```python
from build123d import *

# Parameters (mm, degrees)
F0_W     = 19.05
F0_H     = 19.05
F0_W_2   = 12.7
F0_H_2   = 12.7
F1_DEPTH = 136.525
F2_W     = 42.5958
F2_H     = 47.244
F3_DEPTH = 9.525
F4_R     = 6.35
F5_R     = 1.5875


with BuildPart() as f1:
    # F0 (on Front) → F1 (new body)
    with BuildSketch(Plane.XZ):
        with Locations((68.0290833116, -52.153282702)):
            Rectangle(F0_W, F0_H)
        with Locations((68.0290833116, -52.153282702)):
            Rectangle(F0_W_2, F0_H_2, mode=Mode.SUBTRACT)
    extrude(amount=-F1_DEPTH)

    # F2 (on face) → F3 (join)
    with BuildSketch(Plane.XY.offset(-42.628282702)):
        with Locations((68.0290833116, 68.2625)):
            Rectangle(F2_W, F2_H)
    extrude(amount=F3_DEPTH)

    # F4
    f4_edges = [f1.edges().sort_by_distance(p)[0] for p in [
        (89.326983, 44.6405, -37.865783),
        (89.326983, 91.8845, -37.865783),
        (46.731183, 44.6405, -37.865783),
        (46.731183, 91.8845, -37.865783),
    ]]
    fillet(f4_edges, radius=F4_R)

    # F5
    f5_edges = [f1.edges().sort_by_distance(p)[0] for p in [
        (77.554083, 68.2625, -61.678283),
        (58.504083, 68.2625, -61.678283),
        (58.504083, 22.32025, -42.628283),
        (77.554083, 22.32025, -42.628283),
        (58.504083, 114.20475, -42.628283),
        (77.554083, 114.20475, -42.628283),
    ]]
    fillet(f5_edges, radius=F5_R)


solid = f1.part
```
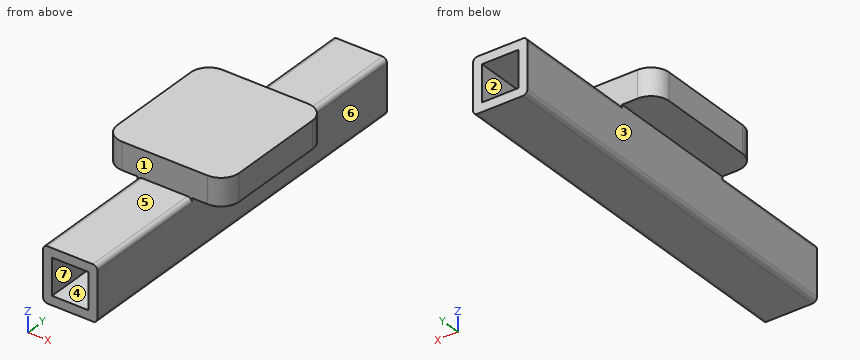
Input: part model. Units: mm. Frame: model coordinates. Face numbers are marked on the shaded views. A direction names the side the tool comes from. Give positions to 0.01 mm unless a question says otherwise; leave off trailing zeros. Order: outer loops, then holes, each group sorted by start corner. A loop starts at its lowest first (then second) coordinate and runs counter-clockwise, first axis right, second up. Notation, with made-up numbers: M -21,-21.5 L 4,-21.5 A21 cw 4,-2.5 Z; hole C 51,83.5 d2. An arc over 180 degrees is marked long. One line per question, with ' | ' between items. Start each with the question number.
1. Section query C-C (y = 124). Return the cut outline in (x, z) (1 decimal), and give its area (3 significant figures).
2. Section query B-B (z = -55.5). Return the cut outline in (x, y) (3 decimals), and give its area (3 significant figures).
3. Section query D-D (y = 61). Return the cut outline in (x, z) (1 decimal).
4. Pull-direction query (X, two-part tool) for the marked faces 1, 2, 3 and 4; classes: released by +X, released by -X, zero draft, split by the parting line, or undercut.
5. Access query for the marked faces 5, 6 and 7. Directions: +Z, -Z, +X, -X, +Y, -Y. A direction counts if a zero-diameter tool reaches every point of the face in a straight line with its end or side. Return the directions, or none.
6. Material intervals for probe 1 along X at (y, z) = (92, -47.75); probe 2 along Z at (x, y) = (64, 23); probe 3 along Z at (x, y) = (63, 70.5), sorted ascending. Write a range as [from, to].
7. Section query A-A (x = 67.5). Return the cut outline in (y, z) (1 decimal).
8. First-contact query: pin 1 Ø6 at (y, z) = (20.5, -44.5) entering from +X; pin 2 Ø2 at (y, z) = (39.5, -48.5) entering from -X; pin 3 Ø5 at (x, y) = (65, 11.5) entering from +Z. Flat tips, straight axial feed; report the tip coordinate or a pass-through.
Here are the results:
1) outline: M 58.5,-60.1 A1.6 ccw 60.1,-61.7 L 76,-61.7 A1.6 ccw 77.6,-60.1 L 77.6,-44.2 A1.6 ccw 76,-42.6 L 60.1,-42.6 A1.6 ccw 58.5,-44.2 Z; hole M 61.7,-58.5 L 74.4,-58.5 L 74.4,-45.8 L 61.7,-45.8 Z | area: 199 mm²
2) outline: M 58.504,0 L 61.679,0 L 61.679,136.525 L 58.504,136.525 Z; M 74.379,0 L 77.554,0 L 77.554,136.525 L 74.379,136.525 Z | area: 867 mm²
3) outline: M 46.7,-42.6 L 58.5,-42.6 L 58.5,-60.1 A1.6 ccw 60.1,-61.7 L 76,-61.7 A1.6 ccw 77.6,-60.1 L 77.6,-42.6 L 89.3,-42.6 L 89.3,-33.1 L 46.7,-33.1 Z; hole M 61.7,-58.5 L 74.4,-58.5 L 74.4,-45.8 L 61.7,-45.8 Z
4) face 1: zero draft | face 2: undercut | face 3: released by -X | face 4: undercut
5) face 5: +Z, +X, -X, -Y | face 6: -Z, +X, +Y, -Y | face 7: +Y, -Y
6) probe 1: [58.5, 61.68], [74.38, 77.55] | probe 2: [-61.68, -58.5], [-45.8, -42.63] | probe 3: [-61.68, -58.5], [-45.8, -33.1]
7) outline: M 0,-61.7 L 136.5,-61.7 L 136.5,-58.5 L 0,-58.5 Z; M 0,-45.8 L 136.5,-45.8 L 136.5,-42.6 L 91.9,-42.6 L 91.9,-33.1 L 44.6,-33.1 L 44.6,-42.6 L 0,-42.6 Z
8) pin 1: x = 77.55 | pin 2: x = 58.5 | pin 3: z = -42.63
